Autodesk Inventor part; units mm, degrees
ref_plane "Work Plane1" through (0, 0, 0) normal (0, 0, 1) x (1, 0, 0)
ref_plane "Work Plane2" through (-23.495, -37.0586, -7.62) normal (0, 0, -1) x (0, 1, 0)
ref_plane "YZ Plane" through (0, 0, 0) normal (1, 0, 0) x (0, 1, 0)
ref_plane "Work Plane1" through (0, 0, 0) normal (0, 0, 1) x (1, 0, 0)
ref_plane "Work Plane2" through (-23.495, -37.0586, -7.62) normal (0, 0, -1) x (0, 1, 0)
sketch "Sketch1" plane through (0, 0, 0) normal (0, 0, 1) x (1, 0, 0)
  circle A0 centre (-14.605, 0) radius 3.81
  line L0 (23.495, -13.6398) -> (23.495, -75.1078)
  line L1 (-14.605, 0) -> (17.145, -54.9926) construction
  circle A1 centre (17.145, -54.9926) radius 3.937
  line L2 (-14.605, 0) -> (17.145, 54.9926) construction
  circle A2 centre (17.145, 54.9926) radius 2.286
  line L3 (19.685, -33.9344) -> (23.495, -33.9344)
  line L4 (19.685, -29.5656) -> (23.495, -29.5656)
  line L5 (23.495, -46.7614) -> (25.0825, -46.7614)
  line L6 (23.495, -72.1614) -> (25.0825, -72.1614)
  line L7 (23.495, -67.5386) -> (25.0825, -67.5386)
  line L8 (23.495, -76.1238) -> (25.0825, -76.1238)
  line L9 (10.1391, -54.1676) -> (16.832, -37.0586)
  line L10 (16.832, -37.0586) -> (16.832, -26.036)
  line L11 (19.685, -27.493) -> (-18.6482, -7.9174)
  line L12 (19.685, -27.493) -> (19.685, -37.0586)
  line L13 (19.685, -37.0586) -> (23.495, -37.0586)
  line L14 (23.495, -37.0586) -> (23.495, -64.1344)
  line L15 (23.495, -64.1344) -> (15.875, -64.1344)
  line L16 (19.685, -64.1344) -> (19.685, -76.1238)
  line L17 (19.685, -76.1238) -> (23.495, -76.1238)
  line L18 (15.875, -64.1344) -> (10.1391, -54.1676)
  line L19 (19.431, -27.3632) -> (19.431, -37.0586)
  line L20 (19.431, -37.0586) -> (19.685, -37.0586)
  line L21 (16.832, -26.2966) -> (19.685, -27.7535)
  line L22 (19.431, -37.0586) -> (19.431, -37.241)
  line L23 (19.431, -37.241) -> (23.495, -37.241)
  line L24 (23.495, -76.1238) -> (23.495, -64.1344)
  circle A3 centre (16.832, -42.2926) radius 2.286
  circle A4 centre (16.832, -67.6926) radius 2.286
  arc A5 (16.832, -37.0586) -> (10.1391, -54.1676) centre (20.3426, -48.2955) ccw
  circle A6 centre (16.832, -67.6926) radius 6.6647
  line L25 (16.832, -74.3574) -> (23.495, -74.3574)
  line L26 (23.495, -76.1238) -> (23.495, -88.8238)
  line L27 (23.495, -88.8238) -> (19.685, -88.8238)
  line L28 (19.685, -88.8238) -> (19.685, -76.1238)
  point P0 (0, 0)
  point P1 (23.495, -37.241)
  point P2 (19.431, -27.6238)
  point P3 (14.3606, -61.503)
  point P4 (19.685, -74.3574)
extrude "Extrusion1" add sketch "Sketch1" against normal up to surface (7.62 mm away) contours L0 L15 A6 L18 L9 A3 L10 L21 L19 L22 L23 | L0 A6 L15 | L9 A3 A5 | L0 A6 L16 L15 | L15 L18 A6 | L0 L25 L16 A6 | L16 A6 L18 L15 | L16 L25 A6 | L0 L24 L17 L16 L25 | L17 L26 L27 L28
sketch "Sketch2" plane through (19.685, -76.1238, 0) normal (-1, 0, 0) x (0, 0, 1)
  circle A0 centre (-3.81, 6.2738) radius 2.1844
  circle A1 centre (-3.81, 44.3738) radius 2.1844
  circle A2 centre (-3.81, 44.3738) radius 2.1844
  circle A3 centre (-3.81, -6.4262) radius 2.1844
  point P0 (0, 76.1238)
  dimension "d22" = 50.8
extrude "Extrusion2" cut sketch "Sketch2" along normal mid plane 25.4 contours A1 | A3
fillet "Fillet1" radius 3.175 2 edges at (14.3606, -61.503, -3.81) (16.832, -37.0586, -3.81)
fillet "Fillet2" radius 3.175 1 edges at (19.685, -74.3574, -3.81)
properties part number "DrivenMotorMount"
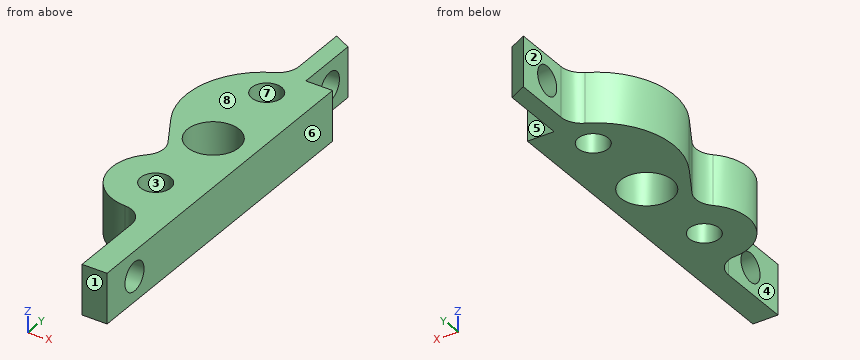
Work out the finished part from the listing and answer in its coordinate system (mm). Face numbers are marked on the shaded views. A direction names the side the tool comes from. Give positions to 0.01 mm unless a question says otherwise; leave off trailing zeros. Write each loop counter-clockwise with the first axis right and the second up, starting at its lowest first coordinate (ties: lowest second). Pieces come first, ordered by that corner, then holes. Notation, with made-up numbers: (-20.5, 42) -> (24.5, 42) arc R17 ccw to (24.5, 59) -> close; hole circle Ø6 at (-36, 83). An arc over 180 degrees is marked (long way). Write each question's results on one line, items separated by ' | '.
1. Each of these flat-tipped pins is pushed along its axis until it touches: pin 1 Ø3.5 at (x, y) = (16.83, -42.29) entering from -Z; pin 2 Ø2.5 at (y, z) = (-33, -5.5) entering from +X; pin 3 Ø1.5 at (x, z) = (15, -1.5) entering from -Y; pin 4 Ø4 at (y, z) = (-43, -4) entering from -X. Where does it stop, or does it pass through?
Data:
pin 1: through | pin 2: x = 19.43 | pin 3: y = -74.27 | pin 4: x = 9.04
2. Find section C-C on z = -3.5. Give the number of separate pieces and of enclosed holes in the cut face, and give its area (3 significant figures).
Data:
separate pieces: 3 | enclosed holes: 3 | area: 441 mm^2
3. A tool of negligible diameter and unlimited length cuts with its end or side. For the marked faces 1, 2, 3, 4 and 5, from which of +Z, -Z, +X, -X, +Y, -Y can it reach the whole face along a straight path? Write none if from no direction.
Data:
face 1: +Z, -Z, +X, -X, -Y | face 2: +Z, -Z, -X, +Y | face 3: +Z, -Z | face 4: +Z, -Z, -X, -Y | face 5: +Z, -Z, +X, +Y
4. Determine the mould class of the marked faces 6, 7 and 8 for opening direction X: +X half, -X half, draft (parallel to the pull), parting line (faces both ways), or undercut.
Data:
face 6: +X half | face 7: undercut | face 8: draft
5. Find section A-A on y = -82.55. Determine the outline of the cut face in (x, z) (3 decimals).
Data:
outline: (19.685, -7.62) -> (23.495, -7.62) -> (23.495, -5.994) -> (19.685, -5.994) -> close; (19.685, -1.626) -> (23.495, -1.626) -> (23.495, 0) -> (19.685, 0) -> close
6. Find section D-D on y = -31.75. Determine the outline of the cut face in (x, z).
Data:
outline: (16.83, -7.62) -> (19.43, -7.62) -> (19.43, -5.99) -> (16.83, -5.99) -> close; (16.83, -1.63) -> (19.43, -1.63) -> (19.43, 0) -> (16.83, 0) -> close
7. Find section B-B on x = 15.75. Determine the outline of the cut face in (y, z).
Data:
outline: (-74.27, -7.62) -> (-69.71, -7.62) -> (-69.71, 0) -> (-74.27, 0) -> close; (-65.68, -7.62) -> (-58.67, -7.62) -> (-58.67, 0) -> (-65.68, 0) -> close; (-51.31, -7.62) -> (-44.31, -7.62) -> (-44.31, 0) -> (-51.31, 0) -> close; (-40.28, -7.62) -> (-37.31, -7.62) -> (-37.31, 0) -> (-40.28, 0) -> close
8. Straight lines are drawn through the part: L1, parallel to Z at x = 18.75, y = -31.75; L2, parallel to Y at x = 15.25, z = -1.5; L3, parallel to Y at x = 18.75, z = -2.75. For each, find the intervals that lie inside material, in ascending order.
Data:
L1: -7.62 to -5.99, -1.63 to 0 | L2: -74.17 to -69.34, -66.04 to -58.44, -51.54 to -43.94, -40.64 to -37.67 | L3: -75.28 to -68.94, -66.45 to -58.59, -51.4 to -43.54, -41.05 to -33.66, -29.84 to -27.28
